```python
from build123d import *

# Parameters (mm, degrees)
F1_DEPTH = 25.4
F2_DEPTH = 25.4
F3_DEPTH = 9.525
F4_DEPTH = 9.525
F5_DEPTH = 15.875
F6_DEPTH = 15.875


with BuildPart() as f1:
    # F0 (on Front) → F1 (new body)
    with BuildSketch(Plane.XZ):
        with BuildLine():
            Line((0, 25.4), (0, 42.8625))
            ThreePointArc((0, 42.8625), (-42.8625, 0), (0, -42.8625))
            Line((0, -42.8625), (0, -25.4))
            ThreePointArc((0, -25.4), (-25.4, 0), (0, 25.4))
        make_face()
        with BuildLine():
            Line((4.499378453, 42.6256906077), (0, 42.8625))
            Line((0, 42.8625), (0, 25.4))
            ThreePointArc((0, 25.4), (17.9605122421, 17.9605122421), (25.4, 0))
            Line((25.4, 0), (42.8625, 0))
            ThreePointArc((42.8625, 0), (31.8594453435, 28.6735008092), (4.499378453, 42.6256906077))
        make_face()
        with BuildLine():
            Line((0, -25.4), (0, -42.8625))
            Line((0, -42.8625), (4.499378453, -42.6256906077))
            ThreePointArc((4.499378453, -42.6256906077), (31.8594453435, -28.6735008092), (42.8625, 0))
            Line((42.8625, 0), (25.4, 0))
            ThreePointArc((25.4, 0), (17.9605122421, -17.9605122421), (0, -25.4))
        make_face()
    extrude(amount=F1_DEPTH)

    # F2 (add): a face of the model
    f2_faces = [f1.faces().sort_by_distance(p)[0] for p in [
        (-41.6501654237, 0, 0),
    ]]
    extrude(f2_faces, amount=F2_DEPTH)

    # F0 (on Front) → F3 (join)
    with BuildSketch(Plane.XZ):
        with BuildLine():
            Line((0, -25.4), (0, -42.8625))
            Line((0, -42.8625), (4.499378453, -42.6256906077))
            ThreePointArc((4.499378453, -42.6256906077), (31.8594453435, -28.6735008092), (42.8625, 0))
            Line((42.8625, 0), (25.4, 0))
            ThreePointArc((25.4, 0), (17.9605122421, -17.9605122421), (0, -25.4))
        make_face()
        with BuildLine():
            Line((180.975, 33.3375), (4.499378453, 42.6256906077))
            ThreePointArc((4.499378453, 42.6256906077), (31.8594453435, 28.6735008092), (42.8625, 0))
            Line((42.8625, 0), (147.6375, 0))
            ThreePointArc((147.6375, 0), (157.4018276822, 23.5731723178), (180.975, 33.3375))
        make_face()
        with BuildLine():
            ThreePointArc((42.8625, 0), (31.8594453435, -28.6735008092), (4.499378453, -42.6256906077))
            Line((4.499378453, -42.6256906077), (180.975, -33.3375))
            ThreePointArc((180.975, -33.3375), (157.4018276822, -23.5731723178), (147.6375, 0))
            Line((147.6375, 0), (42.8625, 0))
        make_face()
    extrude(amount=F3_DEPTH)

    # F0 (on Front) → F4 (join)
    with BuildSketch(Plane.XZ):
        with BuildLine():
            Line((0, 25.4), (0, 42.8625))
            ThreePointArc((0, 42.8625), (-42.8625, 0), (0, -42.8625))
            Line((0, -42.8625), (0, -25.4))
            ThreePointArc((0, -25.4), (-25.4, 0), (0, 25.4))
        make_face()
        with BuildLine():
            Line((4.499378453, 42.6256906077), (0, 42.8625))
            Line((0, 42.8625), (0, 25.4))
            ThreePointArc((0, 25.4), (17.9605122421, 17.9605122421), (25.4, 0))
            Line((25.4, 0), (42.8625, 0))
            ThreePointArc((42.8625, 0), (31.8594453435, 28.6735008092), (4.499378453, 42.6256906077))
        make_face()
        with BuildLine():
            Line((0, -25.4), (0, -42.8625))
            Line((0, -42.8625), (4.499378453, -42.6256906077))
            ThreePointArc((4.499378453, -42.6256906077), (31.8594453435, -28.6735008092), (42.8625, 0))
            Line((42.8625, 0), (25.4, 0))
            ThreePointArc((25.4, 0), (17.9605122421, -17.9605122421), (0, -25.4))
        make_face()
        with BuildLine():
            Line((180.975, 33.3375), (4.499378453, 42.6256906077))
            ThreePointArc((4.499378453, 42.6256906077), (31.8594453435, 28.6735008092), (42.8625, 0))
            Line((42.8625, 0), (147.6375, 0))
            ThreePointArc((147.6375, 0), (157.4018276822, 23.5731723178), (180.975, 33.3375))
        make_face()
        with BuildLine():
            ThreePointArc((42.8625, 0), (31.8594453435, -28.6735008092), (4.499378453, -42.6256906077))
            Line((4.499378453, -42.6256906077), (180.975, -33.3375))
            ThreePointArc((180.975, -33.3375), (157.4018276822, -23.5731723178), (147.6375, 0))
            Line((147.6375, 0), (42.8625, 0))
        make_face()
    extrude(amount=-F4_DEPTH)

    # F0 (on Front) → F5 (join)
    with BuildSketch(Plane.XZ):
        with BuildLine():
            ThreePointArc((147.6375, 0), (157.4018276822, -23.5731723178), (180.975, -33.3375))
            Line((180.975, -33.3375), (180.975, -17.4625))
            ThreePointArc((180.975, -17.4625), (168.6271478335, -12.3478521665), (163.5125, 0))
            Line((163.5125, 0), (147.6375, 0))
        make_face()
        with BuildLine():
            Line((180.975, 17.4625), (180.975, 33.3375))
            ThreePointArc((180.975, 33.3375), (157.4018276822, 23.5731723178), (147.6375, 0))
            Line((147.6375, 0), (163.5125, 0))
            ThreePointArc((163.5125, 0), (168.6271478335, 12.3478521665), (180.975, 17.4625))
        make_face()
        with BuildLine():
            ThreePointArc((214.3125, 0), (204.5481723178, 23.5731723178), (180.975, 33.3375))
            Line((180.975, 33.3375), (180.975, 17.4625))
            ThreePointArc((180.975, 17.4625), (193.3228521665, 12.3478521665), (198.4375, 0))
            ThreePointArc((198.4375, 0), (193.3228521665, -12.3478521665), (180.975, -17.4625))
            Line((180.975, -17.4625), (180.975, -33.3375))
            ThreePointArc((180.975, -33.3375), (204.5481723178, -23.5731723178), (214.3125, 0))
        make_face()
    extrude(amount=F5_DEPTH)

    # F0 (on Front) → F6 (join)
    with BuildSketch(Plane.XZ):
        with BuildLine():
            ThreePointArc((147.6375, 0), (157.4018276822, -23.5731723178), (180.975, -33.3375))
            Line((180.975, -33.3375), (180.975, -17.4625))
            ThreePointArc((180.975, -17.4625), (168.6271478335, -12.3478521665), (163.5125, 0))
            Line((163.5125, 0), (147.6375, 0))
        make_face()
        with BuildLine():
            Line((180.975, 17.4625), (180.975, 33.3375))
            ThreePointArc((180.975, 33.3375), (157.4018276822, 23.5731723178), (147.6375, 0))
            Line((147.6375, 0), (163.5125, 0))
            ThreePointArc((163.5125, 0), (168.6271478335, 12.3478521665), (180.975, 17.4625))
        make_face()
        with BuildLine():
            ThreePointArc((214.3125, 0), (204.5481723178, 23.5731723178), (180.975, 33.3375))
            Line((180.975, 33.3375), (180.975, 17.4625))
            ThreePointArc((180.975, 17.4625), (193.3228521665, 12.3478521665), (198.4375, 0))
            ThreePointArc((198.4375, 0), (193.3228521665, -12.3478521665), (180.975, -17.4625))
            Line((180.975, -17.4625), (180.975, -33.3375))
            ThreePointArc((180.975, -33.3375), (204.5481723178, -23.5731723178), (214.3125, 0))
        make_face()
    extrude(amount=-F6_DEPTH)


solid = f1.part
```
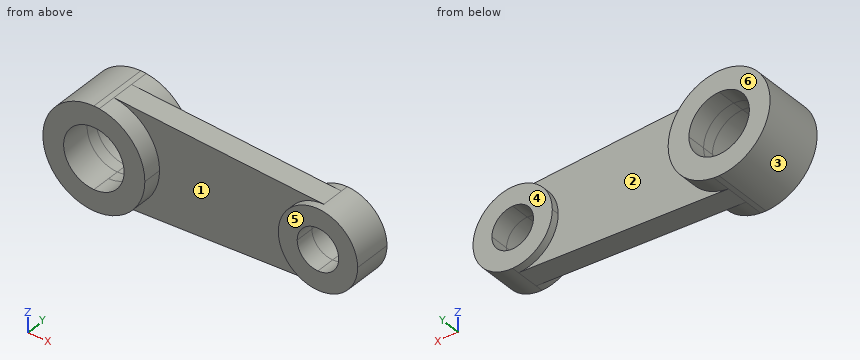
Input: part model. Units: mm. Frame: model coordinates. Face numbers are marked on the shaded views. A direction names the side the tool comes from. Give positions to 0.01 mm unless a question says otherwise; leave off trailing zeros. Loops run counter-clockwise (first coordinate to the right, second up) from the corner with the lowest first, then second, coordinate; pieces in that order, holes last. Notation, with made-up numbers: M -38,-7.75 L -24,-7.75 A26 cw -24,16.25 Z; hole C 75.5,51.5 d11. An arc over 180 degrees is marked long. Answer as CSV lines item,"result". Start each with the question number.
1. Section D-D on x = 21. Return loops of the section in (y, z) (3 decimals), plus the area to 3 significant figures.
2. Pull-direction query (X, two-part tool) for the marked faces 1, 2, 3 and 4; classes: released by +X, released by -X, zero draft, split by the parting line, or undercut.
3. Line query: L1, parallel to X at y = -14.5, z = 17.5; L2, parallel to X at y = 12, z = 19; L3, parallel to X at y = -18.5, z = -17. Output: solid intervals per line, ascending.
4. Section C-C on z = -11.5. Return loops of the section in (x, y) (3 decimals), plus the area to 3 significant figures.
5. Reachability of the marked faces 5 and 6 from +Z, -Z, +X, -X, +Y, -Y: full face, straight path, thin tool, end or side. Return the list, or none.
6. Section B-B on x = -10.5. Return loops of the section in (y, z).
7. Pin query (flat end, axial travel): P1, Ø6, axis at y = 16.5, z = -5, coming from the +X side; P2, Ø5, axis at x = 113, z = -17.5, coming from the +Y side (3 decimals); P3, Ø2, axis at x = 181, y = -12, coming from the +Z side. Return the tip coordinate at first contact, or that it passes through.
8. Section A-A on y = 7. Return loops of the section in (x, z) (1 decimal).
Computed values:
1,outline,"M -25.4,-37.366 L -9.525,-37.366 L -9.525,-41.757 L 9.525,-41.757 L 9.525,-37.366 L 25.4,-37.366 L 25.4,-14.288 L -25.4,-14.288 Z; M -25.4,14.288 L 25.4,14.288 L 25.4,37.366 L 9.525,37.366 L 9.525,41.757 L -9.525,41.757 L -9.525,37.366 L -25.4,37.366 Z"
1,area,"2,510 mm²"
2,face 1,"undercut"
2,face 2,"undercut"
2,face 3,"released by -X"
2,face 4,"zero draft"
3,L1,"x = -39.13 to -18.41, 18.41 to 39.13, 152.6 to 209.35"
3,L2,"x = -38.42 to -16.86, 16.86 to 38.42, 153.58 to 208.37"
3,L3,"x = -39.35 to -18.87, 18.87 to 39.35"
4,outline,"M -41.291,-25.4 L -22.648,-25.4 L -22.648,25.4 L -41.291,25.4 Z; M 22.648,-25.4 L 41.291,-25.4 L 41.291,-9.525 L 149.684,-9.525 L 149.684,-15.875 L 167.834,-15.875 L 167.834,15.875 L 149.684,15.875 L 149.684,9.525 L 41.291,9.525 L 41.291,25.4 L 22.648,25.4 Z; M 194.116,-15.875 L 212.266,-15.875 L 212.266,15.875 L 194.116,15.875 Z"
4,area,"5,110 mm²"
5,face 5,"+Z, -Z, +X, -Y"
5,face 6,"+Z, -Z, +X, -X, +Y"
6,outline,"M -25.4,-41.56 L 25.4,-41.56 L 25.4,-23.13 L -25.4,-23.13 Z; M -25.4,23.13 L 25.4,23.13 L 25.4,41.56 L -25.4,41.56 Z"
7,P1,"stops at x = 214.25"
7,P2,"stops at y = 9.525"
7,P3,"stops at z = 33.34"
8,outline,"M 0,-42.9 L 181,-33.3 A33.3 ccw 181,33.3 L 0,42.9 A42.9 ccw Z; hole C 0,0 d50.8; hole C 181,0 d34.9"
